Design review of the part shown in the three views and the two pictorial views. Dimensions are in mm from the part's minimum x, y and z. Round coordinates to 2 decimals unless told otherwise and drop trailing zeros. Return JSON: item names as keys, results as strings. Group by question number.
1. Take a section at A-A, the plane y = 9.5. Give the number of separate pieces and of enclosed holes in the cut face.
2. Mouldability with a two-part tool opening along X and no side actions: class the marked faces 1, 2, 3 and 4 as pulls with the +X half, pulls with the -X half, needs draft (parallel to the pull), parting line crosses it, or undercut.
3. For line 1 along Y through (x, z) = (37, 2.3) (1 decimal); line 2 along Y through (x, z) = (37.5, 1) (1 decimal); line 3 along X through (y, z) = (0.5, 1.5) (1 decimal), list the stretches that pass through material, from the lowest coordinate up. Write a range as from..to.
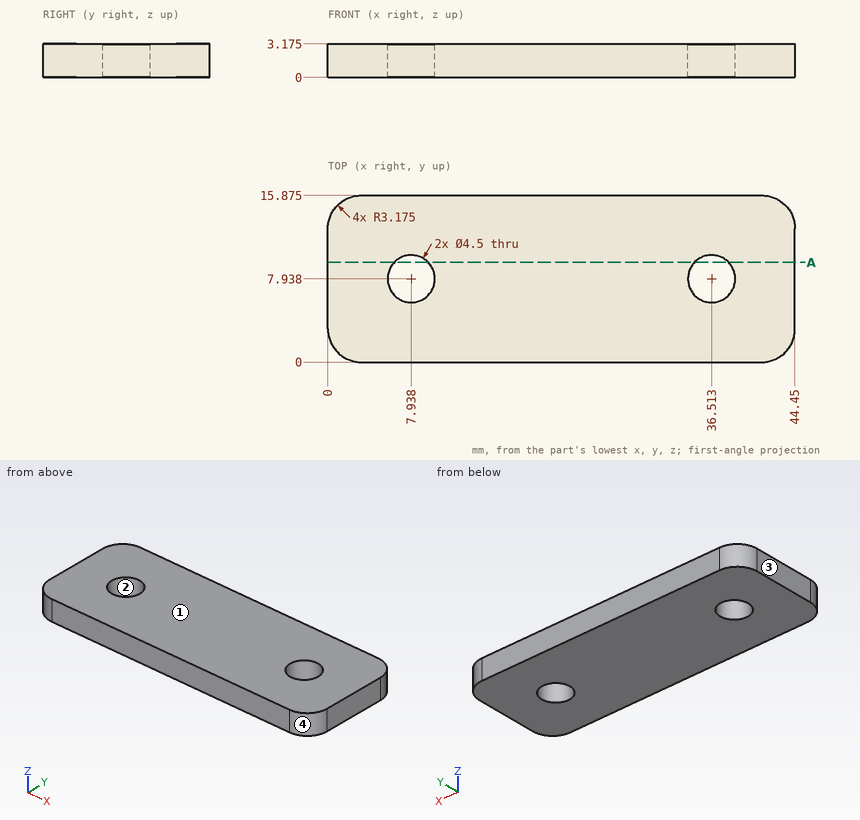
Output:
{
 "1": {"separate pieces": "3", "enclosed holes": "0"},
 "2": {"face 1": "needs draft", "face 2": "undercut", "face 3": "pulls with the -X half", "face 4": "pulls with the +X half"},
 "3": {"line 1": "y = 0..5.7, 10.1..15.9", "line 2": "y = 0..5.9, 10..15.9", "line 3": "x = 1.5..43"}
}
